Here's how the part is built. I have some questions about the finished solid (model axes, mm). Face numbers are marked on the shaded views. A direction names the side the tool comes from. Round coordinates to 2 decimals unless told otherwise and drop trailing zeros. Loops run counter-clockwise (first coordinate to the right, second up) from the corner with the lowest first, then second, coordinate; pieces in that order, holes last. Notation, with made-up numbers: M 15.5,39 L 69.5,39 A20 ccw 69.5,75 Z; hole C 75,89.5 d9. An arc over 180 degrees is marked long. Answer as a JSON object with one key per item and string values.
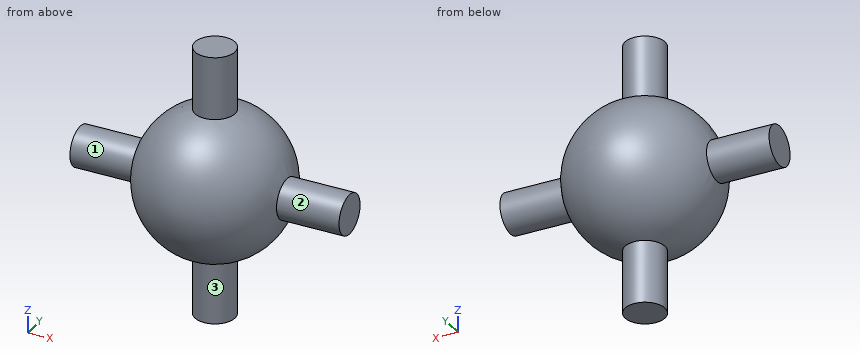
from build123d import *

# Parameters (mm, degrees)
SKETCH2_R           = 1
BOSS_EXTRUDE1_DEPTH = 6.75
CIRPATTERN1_COUNT   = 2
CIRPATTERN1_ANGLE   = 90


with BuildPart() as part:
    # Sketch1 → Revolve2 (revolve)
    with BuildSketch(Plane.XY):
        with BuildLine():
            Line((0, 3.75), (0, -3.75))
            ThreePointArc((0, -3.75), (3.75, 0), (0, 3.75))
        make_face()
    revolve(axis=Axis((0, 3.75, 0), (0, -1, 0)))

    # Sketch2 → Boss-Extrude1 (add, symmetric)
    with BuildSketch(Plane.XY):
        Circle(SKETCH2_R)
    boss_extrude1 = extrude(amount=BOSS_EXTRUDE1_DEPTH, both=True)

    # CirPattern1: Boss-Extrude1 ×2 about axis
    cirpattern1_axis = Axis((0, 4.125, 0), (0, -1, 0))
    for i in range(1, CIRPATTERN1_COUNT):
        add(boss_extrude1.rotate(cirpattern1_axis, i * CIRPATTERN1_ANGLE / (CIRPATTERN1_COUNT - 1)))


solid = part.part
Item 1: I want a section at C-C on x = 0. List the corners of the cut face in (y, z) for me.
Solution:
{"outline": "M -1,-6.75 L 1,-6.75 L 1,-3.61 A3.75 ccw 1,3.61 L 1,6.75 L -1,6.75 L -1,3.61 A3.75 ccw -1,-3.61 Z"}
Item 2: If I drill on L1, parallel to Y at x = 2.5, z = -0.75; L2, parallel to Z at x = -0.25, y = 1; L3, parallel to X at y = -2, z = -0.5, over which ranges is the centre line in solid material (lowest first)? Write a range as from..to.
Solution:
{"L1": "y = -2.69..2.69", "L2": "z = -3.61..3.61", "L3": "x = -3.13..3.13"}
Item 3: I want a section at D-D on y = -0.75. List the corners of the cut face in (x, z) for me, plus the area to 3 significant figures.
Solution:
{"outline": "M -6.75,-0.66 L -3.61,-0.66 A3.67 ccw -0.66,-3.61 L -0.66,-6.75 L 0.66,-6.75 L 0.66,-3.61 A3.67 ccw 3.61,-0.66 L 6.75,-0.66 L 6.75,0.66 L 3.61,0.66 A3.67 ccw 0.66,3.61 L 0.66,6.75 L -0.66,6.75 L -0.66,3.61 A3.67 ccw -3.61,0.66 L -6.75,0.66 Z", "area": "58.8 mm2"}
Item 4: For P1, Ø2, axis at y = -1.5, z = 0, coming from the -X side; P2, Ø8, axis at x = -3, z = 4.5, coming from the -Y side; P3, Ø1, axis at x = 3, y = 2, coming from the +Z side; P4, Ø5, axis at x = -1.5, z = -5.5, coming from the +Y side, each with a flat end and sliding along its axis, tell me the tip position at first contact or that it passes through.
Solution:
{"P1": "stops at x = -6.75", "P2": "stops at y = -3.48", "P3": "stops at z = 2.1", "P4": "stops at y = 1.95"}
Item 5: I want a section at A-A on y = 0. List the corners of the cut face in (x, z) for me, plus the area to 3 significant figures.
Solution:
{"outline": "M -6.75,-1 L -3.61,-1 A3.75 ccw -1,-3.61 L -1,-6.75 L 1,-6.75 L 1,-3.61 A3.75 ccw 3.61,-1 L 6.75,-1 L 6.75,1 L 3.61,1 A3.75 ccw 1,3.61 L 1,6.75 L -1,6.75 L -1,3.61 A3.75 ccw -3.61,1 L -6.75,1 Z", "area": "68.5 mm2"}
Item 6: I want a section at B-B on z = 0. List the corners of the cut face in (x, y) for me, plus the area to 3 significant figures.
Solution:
{"outline": "M -6.75,-1 L -3.61,-1 A3.75 ccw 3.61,-1 L 6.75,-1 L 6.75,1 L 3.61,1 A3.75 ccw -3.61,1 L -6.75,1 Z", "area": "56.4 mm2"}
Item 7: For the marked faces 1, 2 and 3, which set-ups out of +Z, -Z, +X, -X, +Y, -Y let a thin tool reach every point of the face, with its end or its side?
Solution:
{"face 1": "-X", "face 2": "+X", "face 3": "-Z"}
